Read the model definition and answer for the solid it produces. Units are mm, in the model's axes. Round coordinates to 2 decimals unless told otherwise and drop trailing zeros. Write each loop counter-clockwise with the first axis right and the second up, starting at its lowest first coordinate (ties: lowest second). Pieces come first, ordered by that corner, then holes. Notation, with made-up numbers: (21, 52) - (44, 52) arc R31 ccw to (44, 84) - close; hole circle Ø2 at (82, 72.25). An arc over 180 degrees is marked (long way). Use one line per item in the form item = value. Start each with the question number.
1) The part is cut by section C-C, the plane z = -112. Give the vertices of the cut face in (x, y), plus the area to 3 significant figures.
2) The part is cut by section A-A, the plane y = 7. Give the vertices of the cut face in (x, z).
3) The part is cut by section B-B, the plane z = -164.5. Give the vertices of the cut face in (x, y), plus the area to 3 significant figures.
4) Each of these flat-tipped pins is pushed along its axis until it touches: pin 1 (1.5 mm diameter, centred on y = 10.5, z = -93.5, fed in from -X); pin 2 (3.5 mm diameter, centred on x = 44.21, z = -215.53, fed in from -Y); pin 3 (6 mm diameter, centred on x = 166.5, y = 10.5, fed in from +Z); pin 4 (1 mm diameter, centred on x = -82.5, z = -141, fed in from -Y). Where does it stop, or does it pass through?
5) Consider line 1 along X through (y, z) = (4.25, -86); line 2 along X through (y, z) = (2, -132); line 3 along Z through (x, y) = (-162, 6.5). Determine where each line is inside the solid, lowest interval first. Write a range as from..to.
from build123d import *

# Parameters (mm, degrees)
BOSS_EXTRUDE1_DEPTH         = 12.7
TAP_DRILL_FOR_M5X0_8_TAP1_D = 4.2


with BuildPart() as part:
    # Sketch1 → Boss-Extrude1 (new body)
    with BuildSketch(Plane(origin=(0, 0, 0), x_dir=(1, 0, 0), z_dir=(0, 1, 0))):
        Polygon((130.207581625, -225.526146906), (260.415163251, 0), (130.207581625, 225.526146906), (-130.207581625, 225.526146906), (-260.415163251, 0), (-130.207581625, -225.526146906), align=None)
    extrude(amount=BOSS_EXTRUDE1_DEPTH)

    # Tap Drill for M5x0.8 Tap1 (through all)
    with Locations(Plane(origin=(0, 12.7, 0), x_dir=(1, 0, 0), z_dir=(0, 1, 0))):
        with Locations((-44.207581625, 215.526146906), (44.207581625, 215.526146906), (-208.754909213, -69.478184725), (-164.547327587, -146.04796218), (164.547327587, -146.04796218), (208.754909213, -69.478184725)):
            Hole(TAP_DRILL_FOR_M5X0_8_TAP1_D / 2)


solid = part.part
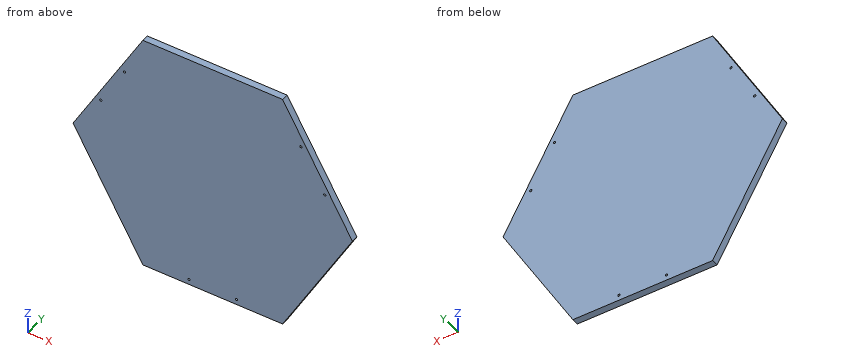
Geometry results:
q1.outline = (-195.75, 0) - (195.75, 0) - (195.75, 12.7) - (-195.75, 12.7) - close
q1.area = 4,970 mm2
q2.outline = (-260.42, 0) - (-130.21, -225.53) - (130.21, -225.53) - (260.42, 0) - (130.21, 225.53) - (-130.21, 225.53) - close; hole circle Ø4.2 at (-208.75, 69.48); hole circle Ø4.2 at (-164.55, 146.05); hole circle Ø4.2 at (-44.21, -215.53); hole circle Ø4.2 at (44.21, -215.53); hole circle Ø4.2 at (164.55, 146.05); hole circle Ø4.2 at (208.75, 69.48)
q3.outline = (-165.44, 0) - (165.44, 0) - (165.44, 12.7) - (-165.44, 12.7) - close
q3.area = 4,200 mm2
q4.pin_1 = -206.87
q4.pin_2 = through
q4.pin_3 = 167.86
q4.pin_4 = 0
q5.line_1 = -210.76..210.76
q5.line_2 = -184.2..184.2
q5.line_3 = -170.46..170.46
